```python
from build123d import *

# Parameters (mm, degrees)
SKETCH_1_R      = 7
SKETCH_1_R_2    = 4.1
EXTRUDE_1_DEPTH = 17
SKETCH_2_R      = 7
EXTRUDE_2_DEPTH = 10
CHAMFER_1_SIZE  = 1
CHAMFER_1_SIZE2 = 1.732050808


with BuildPart() as part:
    # Эскиз1 → Бобышка-Вытянуть1 (new body)
    with BuildSketch(Plane(origin=(0, 0, 0), x_dir=(1, 0, 0), z_dir=(0, 1, 0))):
        with Locations(Location((0, 0, 0), (0, 0, 270))):
            Circle(SKETCH_1_R)
        with Locations(Location((0, 0, 0), (0, 0, 270))):
            Circle(SKETCH_1_R_2, mode=Mode.SUBTRACT)
    extrude(amount=EXTRUDE_1_DEPTH)

    # Эскиз2 → Бобышка-Вытянуть2 (add)
    with BuildSketch(Plane.XZ):
        with Locations(Location((0, 0, 0), (0, 0, 90))):
            Circle(SKETCH_2_R)
    extrude(amount=-EXTRUDE_2_DEPTH)

    # Фаска1
    chamfer_1_edges = [part.edges().sort_by_distance(p)[0] for p in [
        (0, 17, -4.1),
    ]]
    chamfer_1_side = [part.faces().sort_by_distance(p)[0] for p in [
        (0, 17, -6.802010101),
    ]]
    chamfer(chamfer_1_edges, length=CHAMFER_1_SIZE, length2=CHAMFER_1_SIZE2, reference=chamfer_1_side[0])


solid = part.part
```
Part model, mm, in its own coordinate system. Give positions to 0.01 mm unless a question says otherwise; leave off trailing zeros. Order: outer loops, then holes, each group sorted by start corner. A loop starts at its lowest first (then second) coordinate and runs counter-clockwise, first axis right, second up. Notation, with made-up numbers: M 0.25,36.5 L 59.25,36.5 A12 cw 59.25,49.5 Z; hole C -7,23.5 d10. An arc over 180 degrees is marked long. Use a Markdown table: item, result. Add a question column.
(1) Mould opens along Z. For faces 1 (the face through (4.065, 12.597, -0.534)), 2 (the face through (-6.834, 8.381, -1.517)), 3 (the face through (0, 0, 0)), 4 (the face through (0, 10, 0)) say: +Z half, -Z half, draft (parallel to the pull), parting line (faces both ways), or undercut.
(2) Saw through at B-B, the plane z = 0. Give the cut face in (x, y).
(3) Probe line 1 along X through (y, z) = (12.15, 0); line 2 along X through (y, z) = (6.25, 0.25); line 3 along Z through (x, y) = (3, 15.25). List the from-to ranges inside material, lowest first. Write a range as [from, to].
(4) Saw through at C-C, the plane y = 2.25. Give the cut face in (x, z).
(5) Drop flat-ended pins along their axis: P1, Ø2, axis at x = 1.5, z = 0.5, coming from the +Y side; P2, Ø6, axis at y = 4.5, z = 4.5, coming from the +X side. Give the stop position or say it passes through.
(6) Saw through at A-A, the plane x = 0. Give the cut face in (y, z).
(7) Saw through at D-D, the plane x = 6.25. Give the cut face in (y, z), and give its area (3 significant figures).
Answer key:
| question | item | result |
|---|---|---|
| 1 | face 1 | undercut |
| 1 | face 2 | parting line |
| 1 | face 3 | draft |
| 1 | face 4 | undercut |
| 2 | outline | M -7,0 L 7,0 L 7,17 L 5.1,17 L 4.1,15.27 L 4.1,10 L -4.1,10 L -4.1,15.27 L -5.1,17 L -7,17 Z |
| 3 | line 1 | [-7, -4.1], [4.1, 7] |
| 3 | line 2 | [-7, 7] |
| 3 | line 3 | [-6.32, -2.79], [2.79, 6.32] |
| 4 | outline | C 0,0 d14 |
| 5 | P1 | y = 10 |
| 5 | P2 | x = 6.84 |
| 6 | outline | M 0,-7 L 17,-7 L 17,-5.1 L 15.27,-4.1 L 10,-4.1 L 10,4.1 L 15.27,4.1 L 17,5.1 L 17,7 L 0,7 Z |
| 7 | outline | M 0,-3.15 L 17,-3.15 L 17,3.15 L 0,3.15 Z |
| 7 | area | 107 mm^2 |
